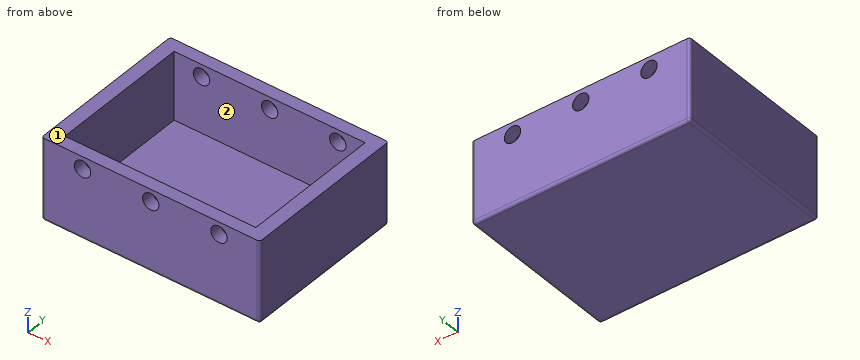
```python
from build123d import *

# Parameters (mm, degrees)
F0_W     = 400
F0_H     = 300
F1_DEPTH = 150
F2_W     = 350
F2_H     = 255
F3_DEPTH = 125
F4_R     = 5
F5_R     = 15
F6_DEPTH = 402


with BuildPart() as f1:
    # F0 (on Top) → F1 (new body)
    with BuildSketch(Plane.XY):
        Rectangle(F0_W, F0_H)
    extrude(amount=F1_DEPTH)

    # F2 (on face) → F3 (cut)
    with BuildSketch(Plane.XY.offset(150)):
        Rectangle(F2_W, F2_H)
    extrude(amount=-F3_DEPTH, mode=Mode.SUBTRACT)

    # F4
    f4_edges = [f1.edges().sort_by_distance(p)[0] for p in [
        (200, 150, 75),
        (200, -150, 75),
        (-200, -150, 75),
        (-200, 0, 0),
        (0, -150, 0),
        (200, 0, 0),
        (0, 150, 0),
        (-200, 150, 75),
    ]]
    fillet(f4_edges, radius=F4_R)

    # F5 (on face) → F6 (cut, symmetric)
    with BuildSketch(Plane(origin=(0, -127.5, 0), x_dir=(-1, 0, 0), z_dir=(0, 1, 0))):
        with Locations((125, 127.5)):
            Circle(F5_R)
        with Locations((-125, 127.5)):
            Circle(F5_R)
        with Locations((0, 127.5)):
            Circle(F5_R)
    extrude(amount=F6_DEPTH, both=True, mode=Mode.SUBTRACT)


solid = f1.part
```
Geometry check sheet. Reference: the model listing, model coordinates, mm. Face numbers are marked on the shaded views. A direction names the side the tool comes from. Round coordinates to 2 decimals unless told otherwise and drop trailing zeros. Write each loop counter-clockwise with the first axis right and the second up, starting at its lowest first coordinate (ties: lowest second). Pieces come first, ordered by that corner, then holes. Notation, with made-up numbers: (-8.75, 84) - (-4.75, 84) arc R27 cw to (-4.75, 105) - close; hole circle Ø1 at (0.5, 58.5). An arc over 180 degrees is marked (long way). Write each question's results on one line, items separated by ' | '.
(1) Sectioned sample at A-A, the plane x = 0. Enter the section's corners in (y, z), plus the area to 3 significant figures.
Computed:
outline: (-150, 5) arc R5 ccw to (-145, 0) - (145, 0) arc R5 ccw to (150, 5) - (150, 112.5) - (127.5, 112.5) - (127.5, 25) - (-127.5, 25) - (-127.5, 112.5) - (-150, 112.5) - close; (-150, 142.5) - (-127.5, 142.5) - (-127.5, 150) - (-150, 150) - close; (127.5, 142.5) - (150, 142.5) - (150, 150) - (127.5, 150) - close | area: 11,800 mm^2
(2) Sectioned sample at B-B, the plane z = 35. Enter the section's corners in (x, y), plus the area to 3 significant figures.
Computed:
outline: (-200, -145) arc R5 ccw to (-195, -150) - (195, -150) arc R5 ccw to (200, -145) - (200, 145) arc R5 ccw to (195, 150) - (-195, 150) arc R5 ccw to (-200, 145) - close; hole (-175, -127.5) - (175, -127.5) - (175, 127.5) - (-175, 127.5) - close | area: 30,700 mm^2
(3) Sectioned sample at D-D, the plane x = 67.5. Enter the section's corners in (y, z), plus the area to 3 significant figures.
Computed:
outline: (-150, 5) arc R5 ccw to (-145, 0) - (145, 0) arc R5 ccw to (150, 5) - (150, 150) - (127.5, 150) - (127.5, 25) - (-127.5, 25) - (-127.5, 150) - (-150, 150) - close | area: 13,100 mm^2
(4) Set-up check for the marked faces 1 and 2: record each of +Z, -Z, +X, -X, +Y, -Y from which the full face is reachable in a straight line by a thin tool's end or side.
Computed:
face 1: +Z, +X, -X, +Y, -Y | face 2: +Z
(5) Thickness scan on probe 1 along X at (y, z) = (-133, 127); probe 2 along X at (y, z) = (116.5, 30.5); probe 3 along Z at (x, y) = (-125, 133). Record the ranges inside material, lowest first. Write a range as from..to.
Computed:
probe 1: x = -200..-139.99, -110.01..-14.99, 14.99..110.01, 139.99..200 | probe 2: x = -200..-175, 175..200 | probe 3: z = 0..112.5, 142.5..150
(6) Depth check by flat-ended pin: pin 1 Ø18 at (x, z) = (-125, 127.5) entering from -Y; pin 2 Ø3 at (x, y) = (71, 96) entering from +Z. Enter the tip coordinate at first touch or a pass-through.
Computed:
pin 1: passes through | pin 2: stops at z = 25
(7) Sectioned sample at C-C, the plane y = 121. Enter the section's corners in (x, z), plus the area to 3 significant figures.
Computed:
outline: (-200, 5) arc R5 ccw to (-195, 0) - (195, 0) arc R5 ccw to (200, 5) - (200, 150) - (175, 150) - (175, 25) - (-175, 25) - (-175, 150) - (-200, 150) - close | area: 16,200 mm^2
